from build123d import *

# Parameters (mm, degrees)
F0_R     = 15
F1_DEPTH = 120
F0_W     = 185
F0_H     = 155
F0_R_2   = 8.5
F2_DEPTH = 5


with BuildPart() as f1:
    # F0 (on Front) → F1 (new body)
    with BuildSketch(Plane.XZ):
        Circle(F0_R)
    extrude(amount=F1_DEPTH)

    # F0 (on Front) → F2 (join)
    with BuildSketch(Plane.XZ):
        Rectangle(F0_W, F0_H)
        with Locations((-61.25, 0)):
            Circle(F0_R_2, mode=Mode.SUBTRACT)
        Circle(F0_R, mode=Mode.SUBTRACT)
        with Locations((61.25, 0)):
            Circle(F0_R_2, mode=Mode.SUBTRACT)
    extrude(amount=F2_DEPTH)


solid = f1.part
The listing builds one solid part. Answer for the finished solid, in the listing's coordinates (mm). A direction names the side the tool comes from. Round coordinates to 2 decimals unless told otherwise and drop trailing zeros. Order: outer loops, then holes, each group sorted by start corner. A loop starts at its lowest first (then second) coordinate and runs counter-clockwise, first axis right, second up. Notation, with made-up numbers: M 58,-25 L 83,-25 A21 cw 83,9 Z; hole C 59,-26.5 d9. An arc over 180 degrees is marked long. Answer in a Markdown table with one row per item. Add a question column.
1) The part is cut by section D-D on y = -69. Determine the outline of the cut face in (x, z).
2) Consider line 1 along Z through (x, y) = (61, -3); line 2 along Y through (x, z) = (28, -67.5); line 3 along Z through (x, y) = (0.5, -75). Determine where each line is inside the solid, lowest interval first. Write a range as from..to.
3) The part is cut by section C-C on x = 0. Determine the outline of the cut face in (y, z), plus the area to 4 significant figures.
4) Determine the mould class of faces 1 (the face through (0, -120, 0)), 2 (the face through (52.76, -2.46, 0.37)), 3 (the face through (92.5, -2, -1)) for opening direction X: pulls with the +X half, pulls with the -X half, needs draft (parallel to the pull), parting line crosses it, or undercut.
5) Which of the six approach directions +Z, -Z, +X, -X, +Y, -Y give full straight-line access (tool end or side, diameter ignored) to faces 4 (the face through (-69.74, -2.46, 0.37)), 5 (the face through (-14.985, -61.695, 0.66))?
6) Flat-ended cylindrical pins translate along their axes: pin 1 Ø22 at (x, z) = (61.25, 0) entering from +Y; pin 2 Ø5 at (y, z) = (-80.5, 16) entering from -X; pin 3 Ø5 at (y, z) = (-42, -16) entering from +X; pin 4 Ø10 at (y, z) = (-95, -2) entering from -X. Find the tip coordinate at first contact, or state that the pin passes through.
7) The part is cut by section B-B on x = 61.25. Determine the outline of the cut face in (y, z).
8) The part is cut by section A-A on z = 0. Determine the outline of the cut face in (x, y).
Findings below:
| question | item | result |
|---|---|---|
| 1 | outline | C 0,0 d30 |
| 2 | line 1 | z = -77.5..-8.5, 8.5..77.5 |
| 2 | line 2 | y = -5..0 |
| 2 | line 3 | z = -14.99..14.99 |
| 3 | outline | M -120,-15 L -5,-15 L -5,-77.5 L 0,-77.5 L 0,77.5 L -5,77.5 L -5,15 L -120,15 Z |
| 3 | area | 4,225 mm² |
| 4 | face 1 | needs draft |
| 4 | face 2 | undercut |
| 4 | face 3 | pulls with the +X half |
| 5 | face 4 | +Y, -Y |
| 5 | face 5 | -Y |
| 6 | pin 1 | stops at y = 0 |
| 6 | pin 2 | stops at x = -6.54 |
| 6 | pin 3 | stops at x = 6.54 |
| 6 | pin 4 | stops at x = -15 |
| 7 | outline | M -5,-77.5 L 0,-77.5 L 0,-8.5 L -5,-8.5 Z; M -5,8.5 L 0,8.5 L 0,77.5 L -5,77.5 Z |
| 8 | outline | M -92.5,-5 L -69.75,-5 L -69.75,0 L -92.5,0 Z; M -52.75,-5 L -15,-5 L -15,-120 L 15,-120 L 15,-5 L 52.75,-5 L 52.75,0 L -52.75,0 Z; M 69.75,-5 L 92.5,-5 L 92.5,0 L 69.75,0 Z |
